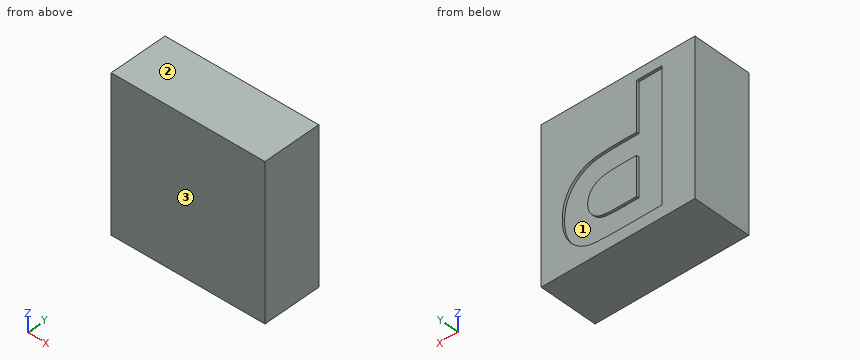
from build123d import *

# Parameters (mm, degrees)
SKETCH1_W           = 31.5
SKETCH1_H           = 31.5
BOSS_EXTRUDE1_DEPTH = 12
CUT_EXTRUDE1_DEPTH  = 0.5


with BuildPart() as part:
    # Sketch1 → Boss-Extrude1 (new body)
    with BuildSketch(Plane(origin=(0, 0, 0), x_dir=(1, 0, 0), z_dir=(0, 1, 0))):
        with Locations((15.75, 15.75)):
            Rectangle(SKETCH1_W, SKETCH1_H)
    extrude(amount=BOSS_EXTRUDE1_DEPTH)

    # Sketch2 → Cut-Extrude1 (cut)
    with BuildSketch(Plane(origin=(0, 12, 0), x_dir=(1, 0, 0), z_dir=(0, 1, 0))):
        with BuildLine():
            Line((6.747621019, 2.065503665), (6.747621019, 29.065503665))
            Line((6.747621019, 29.065503665), (15.385241211, 29.065503665))
            add(Edge.make_bspline(
                [(15.385241211, 29.065503665), (15.776479961, 29.065076414), (16.524770581, 29.064259246), (17.592161888, 29.041554875), (18.553187847, 29.009414336), (19.406422141, 28.969384655), (20.154867078, 28.909652682), (20.795165219, 28.840483957), (21.331348478, 28.766076764), (21.647090916, 28.68907527), (21.789087365, 28.654445973)],
                knots=[0, 0, 0, 0, 1.460485487, 2.793352117, 3.985295279, 5.050041172, 5.981765236, 6.787433016, 7.454681457, 8, 8, 8, 8], degree=3))
            add(Edge.make_bspline(
                [(21.789087365, 28.654445973), (21.977908112, 28.600605902), (22.352673057, 28.493745974), (22.889594358, 28.265937582), (23.40710147, 28.001919809), (23.898692472, 27.687258347), (24.366038435, 27.327539547), (24.810528525, 26.925696963), (25.234533144, 26.479916594), (25.632186734, 25.991079052), (25.996390644, 25.461649309), (26.311154328, 24.890844616), (26.574860483, 24.281145984), (26.799533744, 23.63713522), (26.965298747, 22.951907486), (27.081304113, 22.230223822), (27.162058322, 21.471768579), (27.16777597, 20.952743669), (27.170697942, 20.687498858)],
                knots=[0, 0, 0, 0, 0.907145743, 1.80047177, 2.69161667, 3.591261238, 4.495029544, 5.415863088, 6.359363025, 7.337192411, 8.326890979, 9.326929023, 10.346104993, 11.395420813, 12.477187422, 13.601053412, 14.774031606, 16, 16, 16, 16], degree=3))
            add(Edge.make_bspline(
                [(27.170697942, 20.687498858), (27.162364492, 20.284694456), (27.146322143, 19.509273864), (26.966836725, 18.397614462), (26.693077309, 17.382185261), (26.292958142, 16.472766953), (25.805129757, 15.665790828), (25.267776748, 14.938305662), (24.654198579, 14.312238597), (23.991281493, 13.777486058), (23.290699292, 13.339866766), (22.588848894, 12.966802533), (21.876259855, 12.67997883), (21.390418234, 12.555007436), (21.150866211, 12.493388281)],
                knots=[0, 0, 0, 0, 1.312386234, 2.526415563, 3.661883817, 4.733421185, 5.753802465, 6.732107337, 7.675884281, 8.604170108, 9.50284679, 10.365392406, 11.194030444, 12, 12, 12, 12], degree=3))
            add(Edge.make_bspline(
                [(21.150866211, 12.493388281), (20.979885726, 12.460863774), (20.619479264, 12.392305995), (20.047896175, 12.323966368), (19.423124881, 12.24832185), (18.742595655, 12.198982246), (18.007131761, 12.152777775), (17.217018782, 12.130963119), (16.373385874, 12.104680889), (15.792719174, 12.10420863), (15.493414288, 12.103965204)],
                knots=[0, 0, 0, 0, 0.735353946, 1.55003838, 2.431865514, 3.394945452, 4.432993119, 5.54609699, 6.735134699, 8, 8, 8, 8], degree=3))
            Line((15.493414288, 12.103965204), (11.939928711, 12.103965204))
            Line((11.939928711, 12.103965204), (11.939928711, 2.065503665))
            Line((11.939928711, 2.065503665), (6.747621019, 2.065503665))
        make_face()
        with BuildLine():
            Line((11.939928711, 24.565503665), (11.939928711, 16.603965204))
            Line((11.939928711, 16.603965204), (15.055313327, 16.603965204))
            add(Edge.make_bspline(
                [(15.055313327, 16.603965204), (15.323966729, 16.604313087), (15.837934489, 16.604978632), (16.575364214, 16.628867789), (17.242886299, 16.658028936), (17.841895509, 16.7062966), (18.368776067, 16.769912227), (18.827056361, 16.846004529), (19.217270507, 16.927659519), (19.639233984, 17.062974924), (20.090397304, 17.281902908), (20.572186709, 17.596557411), (20.995438133, 17.97276398), (21.347639417, 18.414605566), (21.628970266, 18.905517169), (21.830403359, 19.440467762), (21.960468518, 20.010591345), (21.972348784, 20.405530729), (21.97839025, 20.60636905)],
                knots=[0, 0, 0, 0, 1.411705958, 2.700771114, 3.876961699, 4.922619712, 5.858038221, 6.66485904, 7.363650596, 7.950905807, 8.989198271, 9.987739806, 10.967313358, 11.951275539, 12.944273208, 13.927870418, 14.946261014, 16, 16, 16, 16], degree=3))
            add(Edge.make_bspline(
                [(21.97839025, 20.60636905), (21.969887549, 20.850986989), (21.953401934, 21.32526892), (21.77161162, 22.000725543), (21.491129938, 22.613710617), (21.090120764, 23.14515141), (20.605711119, 23.592049413), (20.061254895, 23.963884441), (19.445124983, 24.224097423), (19.009070151, 24.324920349), (18.787284481, 24.376200781)],
                knots=[0, 0, 0, 0, 1.085904563, 2.105425768, 3.088705091, 4.068969419, 5.045188284, 6.010769642, 6.988240112, 8, 8, 8, 8], degree=3))
            add(Edge.make_bspline(
                [(18.787284481, 24.376200781), (18.69184504, 24.391465541), (18.479999071, 24.425348577), (18.127867959, 24.460709738), (17.711296797, 24.492870678), (17.229783451, 24.519275772), (16.685236518, 24.53991844), (16.075859838, 24.558006509), (15.40325832, 24.559459645), (14.932712769, 24.563433173), (14.687524865, 24.565503665)],
                knots=[0, 0, 0, 0, 0.564603001, 1.253243608, 2.066786758, 3.005752288, 4.070476343, 5.250658742, 6.567396469, 8, 8, 8, 8], degree=3))
            Line((14.687524865, 24.565503665), (11.939928711, 24.565503665))
        make_face(mode=Mode.SUBTRACT)
    extrude(amount=-CUT_EXTRUDE1_DEPTH, mode=Mode.SUBTRACT)


solid = part.part
For this review, take the finished solid that the model builds, in its own axes (mm). Face numbers are marked on the shaded views. Give positions to 0.01 mm unless a question says otherwise; leave off trailing zeros. Loops run counter-clockwise (first coordinate to the right, second up) from the corner with the lowest first, then second, coordinate; pieces in that order, holes last. Notation, with made-up numbers: (81, 55.25) - (93, 55.25) arc R24 cw to (93, 69.25) - close; hole circle Ø3 at (46.25, 43). An arc over 180 degrees is marked (long way). Write each question's results on one line, items separated by ' | '.
(1) For line 1 along Y through (x, z) = (7, -15), list the stretches that pass through material, from the lowest coordinate up.
Conclusion:
line 1: 0 to 11.5
(2) Draft analysis for pull direction Z (two halves, no side actions). For the marked faces 1, 2 and 3, state which applies: +Z half, -Z half, draft (parallel to the pull), parting line (faces both ways), or undercut.
Conclusion:
face 1: undercut | face 2: +Z half | face 3: draft
(3) Take a section at A-A (x = 11). Give the boundary of the cut face in (y, z).
Conclusion:
outline: (0, -31.5) - (12, -31.5) - (12, -29.07) - (11.5, -29.07) - (11.5, -2.07) - (12, -2.07) - (12, 0) - (0, 0) - close
